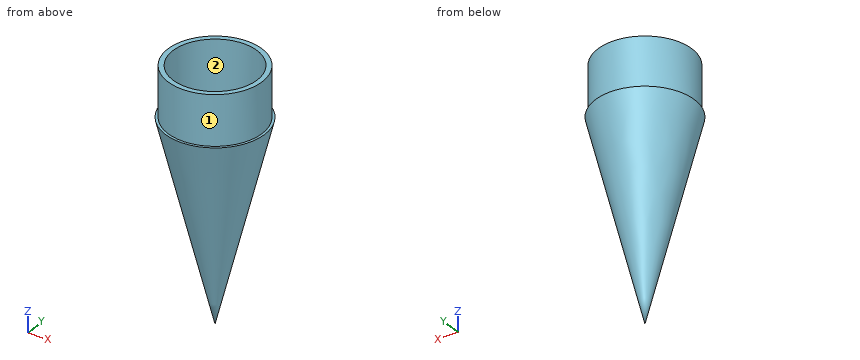
from build123d import *

# Parameters (mm, degrees)
SHELL_1_T = -2


with BuildPart() as part:
    # Эскиз1 → Повернуть1 (revolve)
    with BuildSketch(Plane(origin=(0, 0, 0), x_dir=(1, 0, 0), z_dir=(0, 1, 0)), mode=Mode.PRIVATE) as revolve_1_sk:
        Polygon((0, 80), (-19.9, 0), (-18.9, 0), (-18.9, -20), (-17.643663556, -20), (0, -20), align=None)
    revolve(revolve_1_sk.sketch.rotate(Axis((0, 0, 20), (0, 0, -1)), 180), axis=Axis((0, 0, 20), (0, 0, -1)))

    # Оболочка1
    shell_1_openings = [part.faces().sort_by_distance(p)[0] for p in [
        (0, 0, 20),
    ]]
    offset(amount=SHELL_1_T, openings=shell_1_openings, kind=Kind.INTERSECTION)


solid = part.part
For this review, take the finished solid that the model builds, in its own axes (mm). Face numbers are marked on the shaded views. Give positions to 0.01 mm unless a question says otherwise; leave off trailing zeros. Loops run counter-clockwise (first coordinate to the right, second up) from the corner with the lowest first, then second, coordinate; pieces in that order, holes last. Notation, with made-up numbers: M 24.25,45 L 79.25,45 A10 ccw 79.25,57 Z; hole C 63,89.25 d10. An arc over 180 degrees is marked long. Answer as a JSON object with one key per item and string values. Group by question number.
Q1. Add section B-B on z = -67. Give the boundary of the cut face in (x, y), and give its area (3 significant figures).
Q2. For probe 1 along Y at (x, z) = (0, 4.75); probe 2 along Y at (x, z) = (9, -12.5); probe 3 along X at (y, z) = (11, 4.5), list the stretches that pass through material, from the lowest coordinate up. Write a range as [from, to].
Q3. Add section A-A on z = 2. Give the boundary of the cut face in (x, y).
Q4. Mouldability with a two-part tool opening along X and no side actions: class the marked faces 1 and 2 as +X half, -X half, draft (parallel to the pull), parting line (faces both ways), or undercut.
Q5. Insertion check: P1, Ø12, axis at y = 12, z = -51, coming from the +X side; P2, Ø4, axis at y = 3, z = -62, coming from the +X side; P3, Ø6, axis at y = -16, z = -17.5, coming from the +X side; P4, Ø20, axis at x = 3, y = 6.5, coming from the +Z side. Each pin has a flat end and moves straight along its axis. Give the tip position at first contact, or say it passes through.
Checked values:
{
 "1": {"outline": "C 0,0 d6.47; hole C 0,0 d2.35", "area": "28.5 mm²"},
 "2": {"probe 1": "[-18.9, -16.9], [16.9, 18.9]", "probe 2": "[-14.17, -11.66], [11.66, 14.17]", "probe 3": "[-15.37, -12.83], [12.83, 15.37]"},
 "3": {"outline": "C 0,0 d37.8; hole C 0,0 d33.8"},
 "4": {"face 1": "parting line", "face 2": "undercut"},
 "5": {"P1": "x = 4.39", "P2": "x = 4.57", "P3": "x = 8.72", "P4": "z = 20"}
}
